Work out the finished part from the listing and answer in its coordinate system (mm). Give positions to 0.01 mm unless a question says otherwise; leave off trailing zeros. Loops run counter-clockwise (first coordinate to the right, second up) from the corner with the lowest first, then second, coordinate; pieces in that order, holes last. Notation, with made-up numbers: M 47,-21.5 L 76,-21.5 A9 ccw 76,-16.5 Z; hole C 8,59.25 d2. An arc over 180 degrees is marked long. Answer as a JSON object with one key per item and string values. Group by question number.
```python
from build123d import *

# Parameters (mm, degrees)
F1_DEPTH = 5


with BuildPart() as f1:
    # F0 (on Top) → F1 (new body)
    with BuildSketch(Plane.XY):
        with BuildLine():
            ThreePointArc((50, -10), (40, 0), (50, 10))
            Line((50, 10), (-50, 10))
            ThreePointArc((-50, 10), (-42.9289321881, 7.0710678119), (-40, 0))
            ThreePointArc((-40, 0), (-42.9289321881, -7.0710678119), (-50, -10))
            Line((-50, -10), (50, -10))
        make_face()
        with BuildLine():
            ThreePointArc((60, 0), (57.0710678119, 7.0710678119), (50, 10))
            Line((50, 10), (50, -10))
            ThreePointArc((50, -10), (57.0710678119, -7.0710678119), (60, 0))
        make_face()
        with BuildLine():
            Line((50, -10), (50, 10))
            ThreePointArc((50, 10), (40, 0), (50, -10))
        make_face()
        with BuildLine():
            ThreePointArc((-40, 0), (-42.9289321881, 7.0710678119), (-50, 10))
            Line((-50, 10), (-50, -10))
            ThreePointArc((-50, -10), (-42.9289321881, -7.0710678119), (-40, 0))
        make_face()
        with BuildLine():
            Line((-50, -10), (-50, 10))
            ThreePointArc((-50, 10), (-60, 0), (-50, -10))
        make_face()
    extrude(amount=F1_DEPTH)


solid = f1.part
```
Item 1: Given pin 1 Ø1.5 at (y, z) = (6, 4) entering from +X; pin 2 Ø2 at (y, z) = (-5, 3.5) entering from -X, each flat-ended and moving along its own axis, determine where each tip first touches the part or whether it passes through.
Item 2: Find the intervals of material crossed by probe 1 along X at (y, z) = (8.25, 4.5); probe 2 along X at (y, z) = (-4, 2.2); probe 3 along Y at (x, z) = (-54, 4.7), in increasing order. Write a range as [from, to].
Item 3: A cutting plane is placed at C-C (x = -52). Determine the outline of the cut face in (y, z), and give its area (3 significant figures).
Item 4: A cutting plane is placed at A-A (z = 2.75). Determine the outline of the cut face in (x, y), and give its area (3 significant figures).
Item 5: A cutting plane is placed at B-B (y = -7.25). Determine the outline of the cut face in (x, z).
The answers:
{
 "1": {"pin 1": "stops at x = 58.51", "pin 2": "stops at x = -59.17"},
 "2": {"probe 1": "x = [-55.65, 55.65]", "probe 2": "x = [-59.17, 59.17]", "probe 3": "y = [-9.17, 9.17]"},
 "3": {"outline": "M -9.8,0 L 9.8,0 L 9.8,5 L -9.8,5 Z", "area": "98.0 mm^2"},
 "4": {"outline": "M -50,-10 L 50,-10 A10 ccw 50,10 L -50,10 A10 ccw Z", "area": "2,310 mm^2"},
 "5": {"outline": "M -56.89,0 L 56.89,0 L 56.89,5 L -56.89,5 Z"}
}
